```python
from build123d import *

# Parameters (mm, degrees)
SKETCH2_W               = 120.65
SKETCH2_H               = 9.525
BOSS_EXTRUDE1_DEPTH     = 2.54
SKETCH4_W               = 13.5255
SKETCH4_H               = 1.5875
BOSS_EXTRUDE2_DEPTH     = 120.65
SKETCH13_W              = 120.65
SKETCH13_H              = 2.54
BOSS_EXTRUDE3_DEPTH     = 7.9375
CUT_EXTRUDE4_DEPTH      = 122.664972595
F_6_CLEARANCE_HOLE1_D   = 4.3053
SKETCH15_W              = 1.5875
SKETCH15_H              = 8.4455
SKETCH15_W_2            = 0.79375
BOSS_EXTRUDE4_DEPTH     = 7.9375
CUT_EXTRUDE3_DEPTH      = 122.778845763
CUT_EXTRUDE3_DEPTH_BACK = 122.778845763
SKETCH9_R               = 10.566407632
CUT_EXTRUDE5_REACH      = 123.779
SKETCH16_W              = 3.175
SKETCH16_H              = 4.7625


with BuildPart() as part:
    # Sketch2 → Boss-Extrude1 (new body)
    with BuildSketch(Plane.XY):
        with Locations((60.325, 4.7625)):
            Rectangle(SKETCH2_W, SKETCH2_H)
    extrude(amount=BOSS_EXTRUDE1_DEPTH)

    # Sketch4 → Boss-Extrude2 (add)
    with BuildSketch(Plane.ZY):
        with Locations((6.76275, 0.79375)):
            Rectangle(SKETCH4_W, SKETCH4_H)
    extrude(amount=-BOSS_EXTRUDE2_DEPTH)

    # Sketch13 → Boss-Extrude3 (add)
    with BuildSketch(Plane(origin=(0, 1.5875, 0), x_dir=(1, 0, 0), z_dir=(0, 1, 0))):
        with Locations((60.325, -12.2555)):
            Rectangle(SKETCH13_W, SKETCH13_H)
    extrude(amount=BOSS_EXTRUDE3_DEPTH)

    # Sketch11 → Cut-Extrude4 (cut, through all)
    with BuildSketch(Plane(origin=(0, 1.5875, 0), x_dir=(1, 0, 0), z_dir=(0, 1, 0))):
        with BuildLine():
            Line((63.5, -8.6614), (44.45, -8.6614))
            ThreePointArc((44.45, -8.6614), (42.55135, -6.76275), (44.45, -4.8641))
            Line((44.45, -4.8641), (63.5, -4.8641))
            ThreePointArc((63.5, -4.8641), (65.39865, -6.76275), (63.5, -8.6614))
        make_face()
    extrude(amount=-CUT_EXTRUDE4_DEPTH, mode=Mode.SUBTRACT)

    # #6 Clearance Hole1 (through all)
    with Locations(Plane.XZ):
        with Locations((31.75, 6.76275), (12.7, 6.76275), (107.95, 6.76275)):
            Hole(F_6_CLEARANCE_HOLE1_D / 2)

    # Sketch15 → Boss-Extrude4 (add)
    with BuildSketch(Plane(origin=(0, 1.5875, 0), x_dir=(1, 0, 0), z_dir=(0, 1, 0))):
        with Locations((38.1, -6.76275)):
            Rectangle(SKETCH15_W, SKETCH15_H)
        with Locations((76.2, -6.76275)):
            Rectangle(SKETCH15_W, SKETCH15_H)
        with Locations((120.253125, -6.76275)):
            Rectangle(SKETCH15_W_2, SKETCH15_H)
    extrude(amount=BOSS_EXTRUDE4_DEPTH)

    # Sketch9 → Cut-Extrude3 (cut, two sides: drawn at the far end of the back side and taken through both)
    with BuildSketch(Plane(origin=(0, 0, 0), x_dir=(1, 0, 0), z_dir=(0, 1, 0)).offset(-CUT_EXTRUDE3_DEPTH_BACK)):
        with Locations((-6.35, -2.54)):
            Circle(SKETCH9_R)
    extrude(amount=CUT_EXTRUDE3_DEPTH + CUT_EXTRUDE3_DEPTH_BACK, mode=Mode.SUBTRACT)

    # Sketch16 → Cut-Extrude5 (cut, up to next)
    with BuildSketch(Plane.XY.offset(13.5255), mode=Mode.PRIVATE) as cut_extrude5_sk1:
        with Locations((1.5875, 7.14375)):
            Rectangle(SKETCH16_W, SKETCH16_H)
    cut_extrude5_tool1 = extrude(cut_extrude5_sk1.sketch, amount=-CUT_EXTRUDE5_REACH, mode=Mode.PRIVATE) & part.part
    add(cut_extrude5_tool1.solids().sort_by_distance((1.5875, 7.14375, 13.5255))[0], mode=Mode.SUBTRACT)

    # Mirror1: part across face


with BuildPart() as part_1:
    add(part.part)
    add(part.part.mirror(Plane(origin=(120.65, 4.7625, 6.76275), x_dir=(0, 0, 1), z_dir=(1, 0, 0))))


solid = part_1.part
```
The model under review builds one solid part; all positions refer to its coordinate system, in mm. A direction names the side the tool comes from. Round coordinates to 2 decimals unless told otherwise and drop trailing zeros. Write each loop counter-clockwise with the first axis right and the second up, starting at its lowest first coordinate (ties: lowest second). Pieces come first, ordered by that corner, then holes. Notation, with made-up numbers: (81, 70.25) - (115, 70.25) arc R20 ccw to (115, 92.25) - close; hole circle Ø10 at (37.5, 56). An arc over 180 degrees is marked (long way). Answer as CSV lines item,"result". Start each with the question number.
(1) We need section A-A on x = 133.35. State the section outline as (y, z) points (1 decimal).
(2) To check wall thickness, follow line 1 (X direction, y = 2.5, z = 5); line 2 (Z direction, x = 23.5, y = 8.75); line 3 (Z direction, x = 12.7, y = 0.45). State the ranges of each line that lie inside material, in increasing order.
(3) We need section C-C on x = 58. State the section outline as (y, z) points (1 decimal).
(4) For faces 1 (the flat face through (21, 6, 2.54)), 2 (the cylindrical face through (105.897, 0.805, 7.409)), 3 (the flat face through (223, 1.588, 7)), 4 (the cylindrical face through (4.21, 2.58, 2.12)), 5 (the flat face through (184, 1.588, 4)), list the 3-axis set-ups (+Z, -Z, +X, -X, +Y, -Y) from which the entire face can be reached by the end or side of a thin tool; tool diameter is ignored.
(5) For pin 1 Ø1.5 at (x, z) = (121.5, 5) entering from +Y (3 decimals); pin 2 Ø1 at (y, z) = (4.5, 6.5) entering from -X; pin 3 Ø4 at (y, z) = (7, 5) entering from +X; pin 4 Ø2.5 at (x, z) = (176, 6.5) entering from +Y, all flat-tipped, find the tip position at first contact; note any pin that passes through.
(6) We need section D-D on x = 171. State the section outline as (y, z) points (1 decimal), plus the area to 3 significant figures.
(7) Draft analysis for pull direction Z (two halves, no side actions). For faces 6 (the flat face through (122, 5, 0)), 7 (the cylindrical face through (211.54, 0.8, 5.94)), state which applies: pulls with the +Z half, pulls with the -Z half, needs draft (parallel to the pull), parting line crosses it, or undercut.
(8) We need section B-B on y = 8. Give the number of separate pieces and of enclosed holes in the cut face, plus the area to 3 significant figures.
Worked answers:
1,outline,"(0, 0) - (9.5, 0) - (9.5, 2.5) - (1.6, 2.5) - (1.6, 4.6) - (0, 4.6) - close; (0, 8.9) - (1.6, 8.9) - (1.6, 11) - (9.5, 11) - (9.5, 13.5) - (0, 13.5) - close"
2,line 1,"37.31 to 38.89, 75.41 to 76.99, 119.86 to 121.44, 164.31 to 165.89, 202.41 to 203.99"
2,line 2,"0 to 2.54, 10.99 to 13.53"
2,line 3,"0 to 4.61, 8.92 to 13.53"
3,outline,"(0, 0) - (9.5, 0) - (9.5, 2.5) - (1.6, 2.5) - (1.6, 4.9) - (0, 4.9) - close; (0, 8.7) - (1.6, 8.7) - (1.6, 11) - (9.5, 11) - (9.5, 13.5) - (0, 13.5) - close"
4,face 1,"-X, +Y"
4,face 2,"+Y, -Y"
4,face 3,"+X, +Y"
4,face 4,"-X, +Y, -Y"
4,face 5,"+Y"
5,pin 1,"y = 9.525"
5,pin 2,"x = 37.31"
5,pin 3,"x = 203.99"
5,pin 4,"y = 1.59"
6,outline,"(0, 0) - (9.5, 0) - (9.5, 2.5) - (1.6, 2.5) - (1.6, 11) - (9.5, 11) - (9.5, 13.5) - (0, 13.5) - close"
6,area,"61.8 mm²"
7,face 6,"pulls with the -Z half"
7,face 7,"undercut"
8,separate pieces,"1"
8,enclosed holes,"4"
8,area,"1,260 mm²"
